For this review, take the finished solid that the model builds, in its own axes (mm). A direction names the side the tool comes from. Coordinates: 2 decimals unless noted, no trailing zeros. Loops run counter-clockwise (first coordinate to the right, second up) from the corner with the lowest first, then second, coordinate; pieces in that order, holes last.
```python
from build123d import *

# Parameters (mm, degrees)
SKETCH1_W           = 85
SKETCH1_H           = 85
BOSS_EXTRUDE1_DEPTH = 2
SKETCH2_W           = 85
SKETCH2_H           = 85
SKETCH2_W_2         = 81
SKETCH2_H_2         = 81
BOSS_EXTRUDE2_DEPTH = 43
SKETCH3_R           = 9
CUT_EXTRUDE1_DEPTH  = 2
SKETCH4_W           = 14
SKETCH4_H           = 14
CUT_EXTRUDE2_DEPTH  = 2
FILLET1_R           = 2


with BuildPart() as part:
    # Sketch1 → Boss-Extrude1 (new body)
    with BuildSketch(Plane(origin=(0, 0, 0), x_dir=(1, 0, 0), z_dir=(0, 1, 0))):
        with Locations((5.537676609, -18.97566719)):
            Rectangle(SKETCH1_W, SKETCH1_H)
    extrude(amount=BOSS_EXTRUDE1_DEPTH)

    # Sketch2 → Boss-Extrude2 (add)
    with BuildSketch(Plane(origin=(0, 2, 0), x_dir=(1, 0, 0), z_dir=(0, 1, 0))):
        with Locations((5.537676609, -18.97566719)):
            Rectangle(SKETCH2_W, SKETCH2_H)
        with Locations((5.537676609, -18.97566719)):
            Rectangle(SKETCH2_W_2, SKETCH2_H_2, mode=Mode.SUBTRACT)
    extrude(amount=BOSS_EXTRUDE2_DEPTH)

    # Sketch3 → Cut-Extrude1 (cut)
    with BuildSketch(Plane.XY.offset(61.47566719)):
        with Locations((-7.962323391, 15)):
            Circle(SKETCH3_R)
        with Locations((19.037676609, 15)):
            Circle(SKETCH3_R)
    extrude(amount=-CUT_EXTRUDE1_DEPTH, mode=Mode.SUBTRACT)

    # Sketch4 → Cut-Extrude2 (cut)
    with BuildSketch(Plane(origin=(48.037676609, 0, 0), x_dir=(0, 0, -1), z_dir=(1, 0, 0))):
        with Locations((-16.47566719, 9)):
            Rectangle(SKETCH4_W, SKETCH4_H)
    extrude(amount=-CUT_EXTRUDE2_DEPTH, mode=Mode.SUBTRACT)

    # Fillet1
    fillet1_edges = [part.edges().sort_by_distance(p)[0] for p in [
        (47.037676609, 2, 23.47566719),
        (47.037676609, 16, 23.47566719),
        (47.037676609, 16, 9.47566719),
        (47.037676609, 2, 9.47566719),
        (-36.962323391, 22.5, -23.52433281),
        (-36.962323391, 22.5, 61.47566719),
        (48.037676609, 22.5, 61.47566719),
        (48.037676609, 22.5, -23.52433281),
    ]]
    fillet(fillet1_edges, radius=FILLET1_R)


solid = part.part
```
Q1. Consider section B-B (y = 30.5). State the section outline as (x, z) points, then the cut area to 3 significant figures.
Q2. For pin 1 Ø24.5 at (x, z) = (4.5, 29.5) entering from +Y; pin 2 Ø11 at (x, y) = (19.04, 15) entering from +Z; pin 3 Ø1.6 at (x, y) = (47, 11.5) entering from -Z, all flat-tipped, find the tip position at first contact; note any pin that passes through.
Q3. Wall thickness on probe 1 along Z at (x, y) = (-17.5, 20); probe 2 along X at (y, z) = (43.5, -5.5); probe 3 along Y at (x, z) = (-21, 34.5): over which ranges is each line inside the solid? List them lowest first.
Q4. Machinability: for faces 1 (the face through (12.4, 21.08, 60.49)), 2 (the face through (46.038, 23, 20)), 3 (the face through (47, 16, 17)), which of the approach directions +Z, -Z, +X, -X, +Y, -Y give a long, thin tool a straight path to every point of the face, cutting with its end or side? Answer none if there is none.
Q5. The part is to be moulded in two halves that separate along Y. For faces 4 (the face through (47.024, 2.601, 22.905)), 5 (the face through (5, 23, -21.524)), 6 (the face through (2, 45, 60)), 7 (the face through (5, 0, 18)), say which applies: +Y half, -Y half, draft (parallel to the pull), parting line (faces both ways), or undercut.
Q6. Consider section A-A (z = 15). State the section outline as (x, y) points, then the cut area to 3 significant figures.
Q7. Consider section C-C (z = -6.5). State the section outline as (x, y) points, then the cut area to 3 significant figures.
Q8. Consider section D-D (x = 29.5). State the section outline as (y, z) points.
Model answer:
1. outline: (-36.96, -21.52) arc R2 ccw to (-34.96, -23.52) - (46.04, -23.52) arc R2 ccw to (48.04, -21.52) - (48.04, 59.48) arc R2 ccw to (46.04, 61.48) - (-34.96, 61.48) arc R2 ccw to (-36.96, 59.48) - close; hole (-34.96, -21.52) - (46.04, -21.52) - (46.04, 59.48) - (-34.96, 59.48) - close
1. area: 661 mm2
2. pin 1: stops at y = 2
2. pin 2: stops at z = -21.52
2. pin 3: stops at z = -23.52
3. probe 1: z = -23.52 to -21.52, 59.48 to 61.48
3. probe 2: x = -36.96 to -34.96, 46.04 to 48.04
3. probe 3: y = 0 to 2
4. face 1: +Z
4. face 2: +Y
4. face 3: +X
5. face 4: undercut
5. face 5: draft
5. face 6: +Y half
5. face 7: -Y half
6. outline: (-36.96, 0) - (48.04, 0) - (48.04, 2) - (-34.96, 2) - (-34.96, 45) - (-36.96, 45) - close; (46.04, 16) - (48.04, 16) - (48.04, 45) - (46.04, 45) - close
6. area: 314 mm2
7. outline: (-36.96, 0) - (48.04, 0) - (48.04, 45) - (46.04, 45) - (46.04, 2) - (-34.96, 2) - (-34.96, 45) - (-36.96, 45) - close
7. area: 342 mm2
8. outline: (0, -23.52) - (45, -23.52) - (45, -21.52) - (2, -21.52) - (2, 59.48) - (45, 59.48) - (45, 61.48) - (0, 61.48) - close
